Can you work these out from the model? Positions are in its coordinate system, mm. Face numbers are marked on the shaded views. Round coordinates to 2 decimals unless told otherwise and drop trailing zeros. Order: outer loops, then holes, each group sorted by start corner. A loop starts at its lowest first (then second) coordinate and runs counter-clockwise, first axis right, second up.
from build123d import *

# Parameters (mm, degrees)
F0_R     = 5.334
F1_DEPTH = 25.4


with BuildPart() as f1:
    # F0 (on Top) → F1 (new body)
    with BuildSketch(Plane.XY):
        Polygon((4.912673, 8.509), (-4.912673, 8.509), (-9.825347, 0), (-4.912673, -8.509), (4.912673, -8.509), (9.825347, 0), align=None)
        Circle(F0_R, mode=Mode.SUBTRACT)
        Polygon((9.825347, 8.509), (4.912673, 8.509), (9.825347, 0), align=None)
        Circle(F0_R)
    extrude(amount=F1_DEPTH)

    # F2 (on Front) → F3 (revolve, cut)
    with BuildSketch(Plane.XZ):
        with BuildLine():
            Line((-2.921, 5.08), (-2.921, 0))
            Line((-2.921, 0), (0, 0))
            Line((0, 0), (0, 28.878784))
            Line((0, 28.878784), (-5.334, 28.878784))
            Line((-5.334, 28.878784), (-5.334, 9.543106))
            ThreePointArc((-5.334, 9.543106), (-4.69213, 7.006283), (-2.921, 5.08))
        make_face()
    revolve(axis=Axis((0, 0, 14.439392), (0, 0, -1)), mode=Mode.SUBTRACT)


solid = f1.part
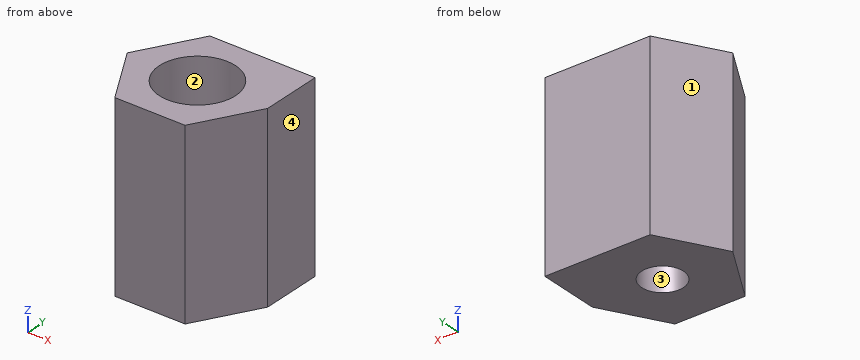
(1) I'm going to push flat-ended pins straight in: pin 1 Ø4 at (x, z) = (-8, 22) entering from -Y; pin 2 Ø3 at (y, z) = (3, 18.5) entering from -X; pin 3 Ø9.5 at (x, y) = (0, 0) entering from +Z. Where does each tip first touch, or does it pass through?
(2) Please list where these lines run through material, in increasing order: probe 1 along Y at (x, z) = (0, 16.75); probe 2 along Y at (x, z) = (0, 1.55); probe 3 along X at (y, z) = (-1.5, 8.5).
(3) If we mould it in two halves opening along X, with no side actions, what happens to the marked faces 1, 2, 3 and 4? For each: pulls with the +X half, pulls with the -X half, needs draft (parallel to the pull), parting line crosses it, or undercut.
(4) I want a section at A-A, the plane z = 10. List the corners of the cut face in (x, y) for me.
(5) I want a section at B-B, the plane y = -6.5. List the corners of the cut face in (x, z) for me.
(6) I want a section at C-C, the plane x = 6.5. List the corners of the cut face in (y, z) for me.
Ans:
1. pin 1: stops at y = -6.63
1. pin 2: stops at x = -8.96
1. pin 3: stops at z = 7.12
2. probe 1: y = -8.51 to -5.33, 5.33 to 8.51
2. probe 2: y = -8.51 to -2.92, 2.92 to 8.51
2. probe 3: x = -8.96 to -5.01, 5.01 to 8.96
3. face 1: pulls with the -X half
3. face 2: undercut
3. face 3: undercut
3. face 4: pulls with the +X half
4. outline: (-9.83, 0) - (-4.91, -8.51) - (4.91, -8.51) - (9.83, 0) - (9.83, 8.51) - (-4.91, 8.51) - close; hole circle Ø10.67 at (0, 0)
5. outline: (-6.07, 0) - (6.07, 0) - (6.07, 25.4) - (-6.07, 25.4) - close
6. outline: (-5.76, 0) - (8.51, 0) - (8.51, 25.4) - (-5.76, 25.4) - close
